The model under review builds one solid part; all positions refer to its coordinate system, in mm. Face numbers are marked on the shaded views. Round coordinates to 2 decimals unless told otherwise and drop trailing zeros. Loops run counter-clockwise (first coordinate to the right, second up) from the corner with the lowest first, then second, coordinate; pieces in that order, holes last. Notation, with made-up numbers: M 1,55.5 L 8,55.5 A23 cw 8,78.5 Z; hole C -13,-38.75 d10. An arc over 180 degrees is marked long. One line per question, with ' | ' between items.
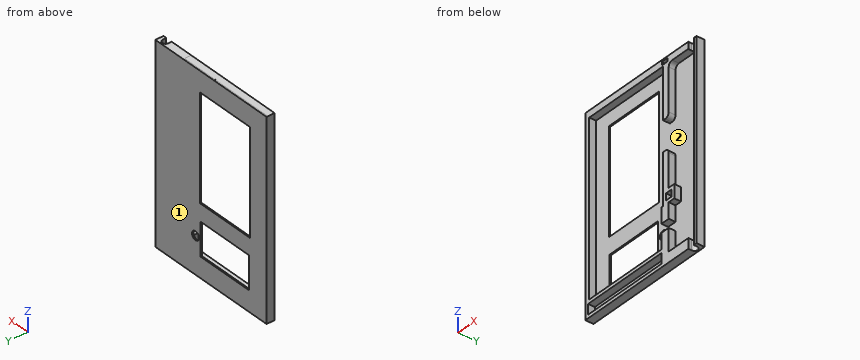
Autodesk Inventor part; units mm, degrees
ref_plane "YZ Plane" through (0, 0, 0) normal (1, 0, 0) x (0, 1, 0)
ref_plane "XZ Plane" through (0, 0, 0) normal (0, 1, 0) x (-1, 0, 0)
ref_plane "XY Plane" through (0, 0, 0) normal (0, 0, 1) x (1, 0, 0)
sketch "Sketch1" plane through (0, 0, 0) normal (0, 1, 0) x (-1, 0, 0)
  line L0 (0, 0) -> (0, -194)
  line L1 (0, -194) -> (130, -194)
  line L2 (130, -194) -> (130, 0)
  line L3 (130, 0) -> (0, 0)
  line L4 (0, -194) -> (123.8, -194)
  line L5 (126.866, -194) -> (126.866, -252.6)
  line L6 (126.866, -252.6) -> (3.066, -252.6)
  line L7 (3.066, -252.6) -> (3.066, -194)
  line L8 (140, 0) -> (140, -262.6)
  line L9 (140, -262.6) -> (0, -262.6)
  line L10 (140, 0) -> (140, 10)
  line L11 (-10, 0) -> (-10, -262.6)
  line L12 (-10, -262.6) -> (3.066, -262.6)
  line L13 (140, 10) -> (-10, 10)
  line L14 (-10, 10) -> (-10, 0)
  line L15 (-10, 10) -> (-60, 10)
  line L16 (-60, 10) -> (-60, -262.6)
  line L17 (-60, -262.6) -> (-10, -262.6)
  line L18 (108.366, -194) -> (108.366, -247.6)
  line L19 (21.566, -199) -> (21.566, -247.6)
  line L20 (110, -150.1456) -> (110, -20)
  line L21 (110, -174) -> (20, -174)
  line L22 (110, -174) -> (110, -150.1456)
  line L23 (102.8172, -20) -> (110, -20)
  line L24 (102.8172, -20) -> (20, -20)
  line L25 (20, -41.8625) -> (20, -20)
  line L26 (20, -41.8625) -> (20, -174)
  line L27 (21.566, -199) -> (21.566, -200.5)
  line L28 (108.366, -199) -> (21.566, -199)
  line L29 (108.366, -252.6) -> (108.366, -247.6)
  line L30 (108.366, -247.6) -> (21.566, -247.6)
  line L31 (21.566, -194) -> (12.316, -194)
  line L32 (12.316, -217.05) -> (12.316, -223.3)
  circle A0 centre (12.316, -223.3) radius 6.25
  line L33 (130, -194) -> (130, -252.6)
  line L34 (130, -252.6) -> (126.866, -252.6)
  line L35 (0, -194) -> (0, -252.6)
  line L36 (0, -252.6) -> (3.066, -252.6)
  line L37 (102.8172, -247.6) -> (102.8172, -267.6)
  line L38 (102.8172, -267.6) -> (140, -267.6)
  line L39 (140, -267.6) -> (140, -262.6)
  line L40 (102.8172, -267.6) -> (0, -267.6)
  line L41 (0, -267.6) -> (0, -252.6)
  line L42 (130, -252.6) -> (130, -267.6)
  line L43 (126.866, -252.6) -> (126.866, -267.6)
  line L44 (3.066, -252.6) -> (3.066, -267.6)
  line L45 (3.066, -194) -> (3.066, -217)
  line L46 (3.066, -252.6) -> (3.066, -229.6)
  line L47 (3.066, -217) -> (0, -217)
  line L48 (3.066, -229.6) -> (0, -229.6)
  line L49 (0, -217) -> (-10, -217)
  line L50 (0, -229.6) -> (-10, -229.55)
  line L51 (0, -267.6) -> (-60, -267.6)
  line L52 (-60, -267.6) -> (-60, -262.6)
  line L53 (-10, -262.6) -> (-10, -267.6)
  line L54 (-10, -194) -> (-20, -194)
  line L55 (-20, -194) -> (-20, -174)
  line L56 (-20, -174) -> (-10, -174)
  line L57 (-10, 0) -> (-10, -10)
  line L58 (-10, -10) -> (-20, -10)
  line L59 (-20, -10) -> (-20, 0)
  line L60 (37.3032, -247.6) -> (37.3032, -277.6)
  line L61 (37.3032, -277.6) -> (-60, -277.6)
  line L62 (-60, -277.6) -> (-60, -267.6)
  line L63 (140, -267.6) -> (140, -277.6)
  line L64 (140, -277.6) -> (37.3032, -277.6)
  dimension "d18" = 12.5
  dimension "d0" = 194
  dimension "d1" = 130
  dimension "d2" = 123.8
  dimension "d3" = 58.6
  dimension "d4" = 10
  dimension "d5" = 262.6
  dimension "d6" = 10
  dimension "d7" = 10
  dimension "d8" = 50
  dimension "d14" = 6.5
  dimension "d15" = 5
  dimension "d16" = 5
  dimension "d17" = 9.25
  dimension "d19" = 20
  dimension "d29" = 23
  dimension "d30" = 23
  dimension "d46" = 10
  dimension "d47" = 10
  dimension "d55" = 30
sketch "Sketch2" plane through (0, 0, 0) normal (0, 1, 0) x (-1, 0, 0)
  line L0 (0, 0) -> (0, -194)
  line L1 (0, -194) -> (0, -109)
  line L2 (0, 0) -> (0, -75)
  line L3 (0, -194) -> (0, -119)
  line L4 (0, -119) -> (-10, -119)
  line L5 (-10, -119) -> (-10, -194)
  line L6 (-10, -194) -> (0, -194)
  line L7 (0, -75) -> (-10, -75)
  line L8 (0, 0) -> (-10, 0)
  line L9 (-10, 0) -> (-10, -75)
  line L10 (-10, -262.6) -> (0, -262.6)
  line L11 (0, -262.6) -> (0, -194)
  line L12 (-10, -194) -> (-10, -262.6)
  line L13 (0, -194) -> (0, -262.6)
  line L14 (0, -262.6) -> (3.066, -262.6)
  line L15 (3.066, -262.6) -> (3.066, -252.6)
  line L16 (3.066, -252.6) -> (0, -252.6)
  line L17 (0, -252.6) -> (0, -194)
  line L18 (3.066, -194) -> (3.066, -252.6)
  line L19 (3.066, -252.6) -> (3.066, -224.05)
  line L20 (3.066, -252.6) -> (3.066, -229.6)
  line L21 (3.066, -194) -> (3.066, -217)
  line L22 (3.066, -217) -> (0, -217)
  line L23 (3.066, -229.6) -> (0, -229.6)
  line L24 (0, -217) -> (-10, -217)
  line L25 (0, -229.6) -> (-10, -229.6)
  line L26 (3.066, -252.6) -> (126.866, -252.6)
  line L27 (126.866, -252.6) -> (126.866, -262.6)
  line L28 (126.866, -262.6) -> (3.066, -262.6)
  line L29 (3.066, -252.6) -> (3.066, -262.6)
  line L30 (126.866, -252.6) -> (130, -252.6)
  line L31 (130, -252.6) -> (130, -262.6)
  line L32 (130, -262.6) -> (126.866, -262.6)
  line L33 (130, -252.6) -> (130, 0)
  line L34 (130, 0) -> (0, 0)
  line L35 (130, 0) -> (140, 0)
  line L36 (140, 0) -> (140, -194)
  line L37 (140, -194) -> (140, -252.6)
  line L38 (140, -252.6) -> (130, -252.6)
  line L39 (140, -267.6319) -> (140, -252.6)
  line L40 (140, -267.6319) -> (-10, -267.6319)
  line L41 (-10, -267.6319) -> (-10, -229.6)
  line L42 (-10, 10.006) -> (140, 10.006)
  line L43 (140, 10.006) -> (140, 0)
  line L44 (-10, 10.006) -> (-10, 0)
  line L45 (-10, -75) -> (-10, 0)
  line L46 (0, 0) -> (-10, 0)
  line L47 (0, 0) -> (0, -75)
  line L48 (-10, -75) -> (0, -75)
  line L49 (0, -119) -> (-10, -119)
  line L50 (-10, -194) -> (0, -194)
  line L51 (0, -119) -> (0, -194)
  line L52 (-10, -194) -> (-10, -119)
  line L53 (3.066, -194) -> (0, -194)
  line L54 (3.066, -194) -> (3.066, -217)
  line L55 (-10, -217) -> (3.066, -217)
  line L56 (-10, -217) -> (-10, -194)
  line L57 (-10, -229.6) -> (-10, -267.6319)
  line L58 (3.066, -267.6319) -> (3.066, -229.6)
  line L59 (3.066, -229.6) -> (-9.4866, -229.6)
  line L60 (0, -194) -> (0, 0)
  line L61 (-10, -194) -> (-20, -194)
  line L62 (-20, -194) -> (-20, -184)
  line L63 (-20, -184) -> (-10, -184)
  line L64 (-20, -184) -> (-20, -174)
  line L65 (-20, -174) -> (-10, -174)
  line L66 (-10, -184) -> (-10, -189)
  line L67 (-5, -189) -> (-5, -179)
  line L68 (-5, -179) -> (-15, -179)
  line L69 (-15, -179) -> (-15, -189)
  line L70 (-15, -189) -> (-5, -189)
  line L71 (0, 0) -> (0, 2.5)
  line L72 (0, 2.5) -> (-7.5, 2.5)
  line L73 (-7.5, 2.5) -> (-7.5, 7.5)
  line L74 (-7.5, 7.5) -> (0, 7.5)
  line L75 (0, 7.5) -> (2.5, 7.5)
  line L76 (2.5, 7.5) -> (2.5, 2.5)
  line L77 (2.5, 2.5) -> (0, 2.5)
  line L78 (-10, -282.6) -> (-10, -267.6319)
  line L79 (50.7455, -277.6) -> (-5, -277.6)
  line L80 (-5, -277.6) -> (-5, -257.6)
  line L81 (-5, -257.6) -> (50.7455, -257.6)
  line L82 (50.7455, -257.6) -> (135, -257.6)
  line L83 (135, -257.6) -> (135, -277.6)
  line L84 (135, -277.6) -> (50.7455, -277.6)
  line L85 (140, -277.6) -> (-60, -277.6)
  line L86 (-60, -277.6) -> (-60, -262.6)
  line L87 (-10, -262.6) -> (-60, -262.6)
  line L88 (140, -277.6) -> (140, -267.6319)
  line L89 (3.066, -267.6319) -> (3.066, -272.6159)
  line L90 (3.066, -272.6159) -> (135, -272.6159)
  line L91 (130, -252.6) -> (133, -252.6)
  line L92 (133, -252.6) -> (133, 0)
  line L93 (133, 0) -> (130, 0)
  point P0 (-10, -277.6)
  point P1 (135, -267.6319)
  point P2 (-5, -267.6319)
  point P3 (3.066, -257.6)
  dimension "d22" = 75
  dimension "d23" = 75
  dimension "d24" = 10
  dimension "d25" = 262.6
  dimension "d27" = 23
  dimension "d28" = 23
  dimension "d48" = 10
  dimension "d49" = 10
  dimension "d50" = 10
  dimension "d51" = 2.5
  dimension "d52" = 7.5
  dimension "d53" = 5
  dimension "d54" = 2.5
  dimension "d67" = 3
extrude "Extrusion1" add sketch "Sketch2" against normal blind 10 contours L0 L7 L9 L8 | L8 L44 L42 L43 L35 L34 | L31 L82 L27 L30 | L38 L39 L40 L83 L82 L31 | L35 L36 L37 L38 L92 | L0 L6 L5 L70 L67 L68 L4 | L27 L82 L81 L15 L26 | L11 L24 L12 L6 | L53 L18 L22 L11 | L15 L81 L11 L16 | L16 L11 L23 L18 | L61 L62 L63 L69 L70 L5 | L5 L68 L69 L63 L64 L65 | L15 L14 L11 L81 | L11 L81 L80 L10 L12 L25 | L40 L88 L85 L83 | L58 L40 L80 L10 L14 | L11 L10 L80 L81 | L89 L90 L83 L84 L79 L80 L40 | L80 L85 L78 L40 | L40 L41 L10 L80 | L41 L78 L85 L86 L87
extrude "Extrusion2" add sketch "Sketch1" along normal blind 2 contours L3 L2 L1 L0 | L0 L35 L49 L11 L14 L13 L10 L8 L9 L42 L33 L2 L3 | L1 L7 L47 L35 | L1 L18 L28 L19 L30 L60 L6 L7 | L47 L7 L48 L35 | L35 L50 L11 L49 | L33 L34 L5 L1 | L48 L7 L36 L35 | L35 L41 L12 L11 L50 | L11 L17 L16 L15 L14 L56 L55 L54 | L5 L6 L29 L18 L1 | L42 L9 L43 L34 | L36 L44 L9 L41 | L54 L55 L56 L11 | L43 L9 L37 L6 | L42 L38 L43 L9 | L9 L39 L38 L42 | L6 L60 L9 L44 | L41 L51 L53 L12 | L9 L44 L40 L41 | L53 L51 L52 L17 | L6 L37 L30 L29 | L43 L38 L37 L9 | L38 L63 L64 L60 L40 | L60 L30 L37 L6 | L6 L37 L9 L60 | L9 L60 L40 L44 | L40 L60 L61 L62 L51 | L37 L40 L60 L9
sketch "Sketch3" plane through (0, 0, 0) normal (0, -1, 0) x (1, 0, 0)
  line L0 (10, -262.6) -> (10, -194)
  line L1 (60, -267.6) -> (-140, -267.6)
  line L2 (10, -267.6319) -> (60, -267.6)
  line L3 (60, 10) -> (60, -267.6)
  line L4 (60, -267.6) -> (60, 10)
  line L5 (10, 10) -> (10, -75)
  line L6 (60, 10) -> (10, 10)
  line L7 (10, 10) -> (10, 0)
  line L8 (10, 0) -> (60, 0)
  line L9 (60, 0) -> (50, 0)
  line L10 (50, 0) -> (50.1707, -267.6063)
  line L11 (50.1707, -267.6063) -> (50.1643, -257.6063)
  line L12 (50.1643, -257.6063) -> (10, -257.6319)
  line L13 (50.1643, -257.6063) -> (60, -257.6063)
  point P0 (0, 0)
  point P1 (10, -229.6)
  point P2 (10, -267.6)
  point P3 (50.1707, -267.6)
  dimension "d35" = 10
  dimension "d36" = 10
extrude "Extrusion3" add sketch "Sketch3" along normal blind 10
fillet "Fillet2" radius 6.25 4 edges at (10, -5, -75) (10, -5, -119) (10, -5, 0) (50, -5, 0)
fillet "Fillet3" radius 1.25 1 edges at (-3.066, -5, -194)
sketch "Sketch8" plane through (-140, 2, 10) normal (0, 0, 1) x (1, 0, 0)
  line L0 (190.1675, -12) -> (190.1675, -2)
  circle A0 centre (190.1675, -7) radius 4.8934
  line L1 (185.2741, -7) -> (185.2741, -11.8934)
  line L2 (185.2741, -11.8934) -> (195.0609, -11.8934)
  line L3 (195.0609, -11.8934) -> (195.0609, -7)
  line L4 (185.2741, -11.8934) -> (185.2741, -12.5715)
  line L5 (185.2741, -12.5715) -> (195.0609, -12.5715)
  line L6 (195.0609, -12.5715) -> (195.0609, -11.8934)
  point P0 (140, -2)
extrude "Extrusion7" cut sketch "Sketch8" against normal blind 299.5
sketch "Sketch9" plane through (0, -10, 0) normal (0, -1, 0) x (1, 0, 0)
  line L0 (-135, -272.6159) -> (-135, -257.6)
  line L1 (-135, -272.6159) -> (-135, -257.6)
  line L2 (-135, -257.6) -> (-3.066, -257.6)
  line L3 (-3.066, -257.6) -> (-3.066, -272.6159)
  line L4 (-3.066, -272.6159) -> (-135, -272.6159)
  line L5 (-3.066, -272.6159) -> (-135, -272.6159)
  line L6 (5, -189) -> (15, -189)
  line L7 (5, -179) -> (5, -189)
  line L8 (5, -189) -> (5, -179)
  line L9 (5, -179) -> (15.0244, -179)
  line L10 (15.0244, -179) -> (15.0244, -189)
  line L11 (15.0244, -189) -> (5, -189)
  line L12 (-2.5, 2.5) -> (7.5, 2.5)
  line L13 (-2.5, 7.5) -> (-2.5, 2.5)
  line L14 (-2.5, 2.5) -> (-2.5, 7.5)
  line L15 (5, -189) -> (5, -188.5)
  line L16 (14.5, -188.5) -> (14.5, -179.5)
  line L17 (14.5, -179.5) -> (5.5, -179.5)
  line L18 (5.5, -179.5) -> (5.5, -188.5)
  line L19 (5.5, -188.5) -> (14.5, -188.5)
  line L20 (60, -277.6) -> (-140, -277.6)
  line L21 (-3.566, -271.6357) -> (-3.566, -258.1)
  line L22 (-3.566, -271.6357) -> (-3.566, -272.1159)
  line L23 (-134.5, -271.0768) -> (-134.5, -272.1159)
  line L24 (-134.5, -271.0768) -> (-134.5, -258.1)
  line L25 (-134.5, -272.1159) -> (-3.566, -272.1159)
  line L26 (-3.566, -258.1) -> (-134.5, -258.1)
  line L27 (7.5, 7.5) -> (7.5, 2.5)
  line L28 (7.5, 2.5) -> (7.5, 7.5)
  line L29 (-2.5, 2.5) -> (7.5, 2.5)
  line L30 (7.5, 7.5) -> (-2.5, 7.5)
  line L31 (-2.5, 7.5) -> (-2.5, 7)
  line L32 (-2, 7) -> (7, 7)
  line L33 (-2, 3) -> (-2, 7)
  line L34 (7.5, 7.5) -> (7, 7.5)
  line L35 (7, 7) -> (7, 3)
  line L36 (7.5, 2.5) -> (7.5, 3)
  line L37 (7, 3) -> (-2, 3)
  point P0 (0, 0)
  dimension "d68" = 0.5
  dimension "d69" = 9.5
  dimension "d70" = 9
  dimension "d71" = 9
properties part number "iphone-playbook dock"
1) Add section A-A on x = -50.5. State how many separate pieces and enclosed holes the cut face has, then the cut area to 3 significant figures.
Output values:
separate pieces: 3 | enclosed holes: 0 | area: 370 mm²
2) Add section B-B on z = -223.3. State the section outline as (x, y) points, then the cut area to 3 significant figures.
Output values:
outline: M -140,-10 L -133,-10 L -133,0 L -108.37,0 L -108.37,2 L -140,2 Z; M -21.57,0 L -18.57,0 L -18.57,2 L -21.57,2 Z; M -6.07,0 L 50.14,0 L 50.14,-0.11 A4.89 cw 55.06,-5 L 55.06,-10 L 60,-10 L 60,2 L -6.07,2 Z | area: 326 mm²
3) Mouldability with a two-part tool opening along Z and no side actions: class the marked faces 1 and 2 as +Z half, -Z half, draft (parallel to the pull), parting line (faces both ways), or undercut.
Output values:
face 1: draft | face 2: undercut
4) Insertion check: P1, Ø5, axis at x = 9, z = -185, coming from the -Y side; P2, Ø5, axis at x = 34, y = -0.5, coming from the +Z side. Each pin has a flat end and moves straight along its axis. Give the tip position at first contact, or say it passes through.
Output values:
P1: stops at y = 0 | P2: stops at z = 10
5) For line 1 (X direction, y = -5, z = -11); line 2 (Z direction, x = -114, y = -5.25); line 3 (Z direction, x = -44.5, y = 0.5), list the stretches that pass through material, from the lowest coordinate up.
Output values:
line 1: x = -140 to -133, 0 to 10, 55.06 to 60 | line 2: z = -277.6 to -272.62, -257.6 to -252.6, 0 to 10.01 | line 3: z = -277.6 to -247.6, -199 to -174, -20 to 10
6) Add section C-C on z = -88. State the section outline as (x, y) points.
Output values:
outline: M -140,-10 L -133,-10 L -133,0 L -110,0 L -110,2 L -140,2 Z; M -20,0 L 50.06,0 L 50.06,-0.11 A4.89 cw 55.06,-5 L 55.06,-10 L 60,-10 L 60,2 L -20,2 Z
